Source: three-view drawing plus pictorial views. Frame: mm from the lowest corner of the part. Round coordinates to 2 decimals unless told otherwise and drop trailing zeros. Order: outer loops, then holes, each group sorted by start corner. A loop starts at its lowest first (then second) coordinate and runs counter-clockwise, first axis right, second up. Notation, with made-up numbers: (70, 26) -> (82, 26) arc R21 cw to (82, 42) -> close; hole circle Ø9 at (82.25, -39.5). An arc over 180 degrees is marked (long way). Use a Markdown table: item, result.
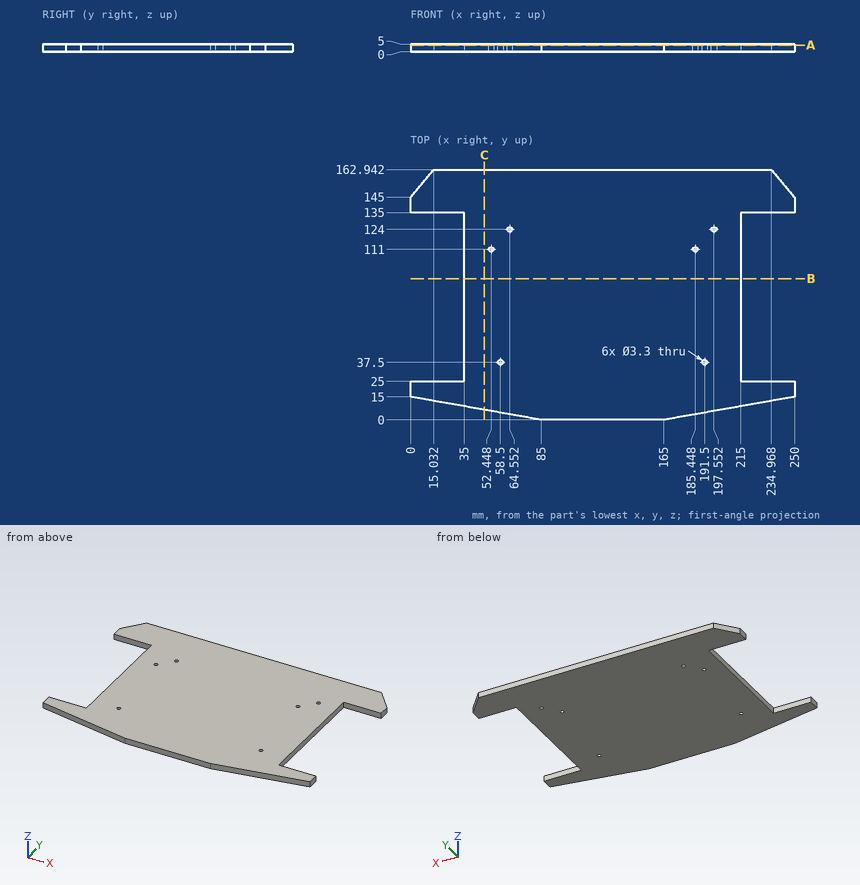
1) Cut plane C-C on x = 48. Return loops of the section in (y, z), and give its area (3 significant figures).
Results found:
| item | result |
|---|---|
| outline | (6.53, 0) -> (162.94, 0) -> (162.94, 5) -> (6.53, 5) -> close |
| area | 782 mm² |
2) Cut plane A-A on z = 4.25. Return loops of the section in (x, y).
Results found:
| item | result |
|---|---|
| outline | (0, 15) -> (85, 0) -> (165, 0) -> (250, 15) -> (250, 25) -> (215, 25) -> (215, 135) -> (250, 135) -> (250, 145) -> (234.97, 162.94) -> (15.03, 162.94) -> (0, 145) -> (0, 135) -> (35, 135) -> (35, 25) -> (0, 25) -> close; hole circle Ø3.3 at (52.45, 111); hole circle Ø3.3 at (58.5, 37.5); hole circle Ø3.3 at (64.55, 124); hole circle Ø3.3 at (185.45, 111); hole circle Ø3.3 at (191.5, 37.5); hole circle Ø3.3 at (197.55, 124) |
3) Cut plane B-B on y = 92. Return loops of the section in (x, z), and give its area (3 significant figures).
Results found:
| item | result |
|---|---|
| outline | (35, 0) -> (215, 0) -> (215, 5) -> (35, 5) -> close |
| area | 900 mm² |
4) Pin query (flat end, axial travel): pin 1 Ø1 at (y, z) = (131.5, 1.5) entering from +X; pin 2 Ø2 at (x, z) = (31, 1.5) entering from -Y; pin 3 Ø1.5 at (x, z) = (10.5, 1.5) entering from -Y (1 decimal). Return the tip coordinate at first contact, or that it passes through.
Results found:
| item | result |
|---|---|
| pin 1 | stops at x = 215 |
| pin 2 | stops at y = 9.35 |
| pin 3 | stops at y = 13 |
5) Line query: L1, parallel to X at y = 37.5, z = 2.6; L2, parallel to X at y = 124, z = 3.8; L3, parallel to X at y = 128.5, z = 2.7. Output: solid intervals per line, ascending. Write a range as [from, to].
Results found:
| item | result |
|---|---|
| L1 | x = [35, 56.85], [60.15, 189.85], [193.15, 215] |
| L2 | x = [35, 62.9], [66.2, 195.9], [199.2, 215] |
| L3 | x = [35, 215] |
